```python
from build123d import *

# Parameters (mm, degrees)
SKETCH1_W           = 60
SKETCH1_H           = 65
BOSS_EXTRUDE1_DEPTH = 21
SKETCH2_W           = 60
SKETCH2_H           = 50
BOSS_EXTRUDE2_DEPTH = 15.25
FILLET1_R           = 5
SKETCH3_R           = 3.25
SKETCH3_R_2         = 1.7
CUT_EXTRUDE4_DEPTH  = 15.25
SKETCH10_R          = 1.7
CUT_EXTRUDE5_DEPTH  = 21


with BuildPart() as part:
    # Sketch1 → Boss-Extrude1 (new body)
    with BuildSketch(Plane.XY):
        with Locations((-22.911585366, 3.368902439)):
            Rectangle(SKETCH1_W, SKETCH1_H)
    extrude(amount=BOSS_EXTRUDE1_DEPTH)

    # Sketch2 → Boss-Extrude2 (add)
    with BuildSketch(Plane.XZ.offset(29.131097561)):
        with Locations((-22.911585366, 46)):
            Rectangle(SKETCH2_W, SKETCH2_H)
    extrude(amount=-BOSS_EXTRUDE2_DEPTH)

    # Fillet1
    fillet1_edges = [part.edges().sort_by_distance(p)[0] for p in [
        (-22.911585366, -13.881097561, 21),
    ]]
    fillet(fillet1_edges, radius=FILLET1_R)

    # Sketch3 → Cut-Extrude4 (cut)
    with BuildSketch(Plane(origin=(0, -13.881097561, 0), x_dir=(1, 0, 0), z_dir=(0, 1, 0))):
        with Locations(Location((-22.911585366, -48.5, 0), (0, 0, 270))):
            Circle(SKETCH3_R)
        with Locations(Location((-11.911585366, -48.5, 0), (0, 0, 270))):
            Circle(SKETCH3_R_2)
        with Locations(Location((-22.911585366, -59.75, 0), (0, 0, 270))):
            Circle(SKETCH3_R_2)
        with Locations(Location((-33.911585366, -48.5, 0), (0, 0, 270))):
            Circle(SKETCH3_R_2)
        with Locations(Location((-22.911585366, -37.5, 0), (0, 0, 270))):
            Circle(SKETCH3_R_2)
    extrude(amount=-CUT_EXTRUDE4_DEPTH, mode=Mode.SUBTRACT)

    # Sketch10 → Cut-Extrude5 (cut)
    with BuildSketch(Plane.XY.offset(21)):
        with Locations((-2.911585366, 25.868902439)):
            Circle(SKETCH10_R)
        with Locations((-2.911585366, 1.118902439)):
            Circle(SKETCH10_R)
        with Locations((-42.911585366, 25.868902439)):
            Circle(SKETCH10_R)
        with Locations((-42.911585366, 1.118902439)):
            Circle(SKETCH10_R)
    extrude(amount=-CUT_EXTRUDE5_DEPTH, mode=Mode.SUBTRACT)


solid = part.part
```
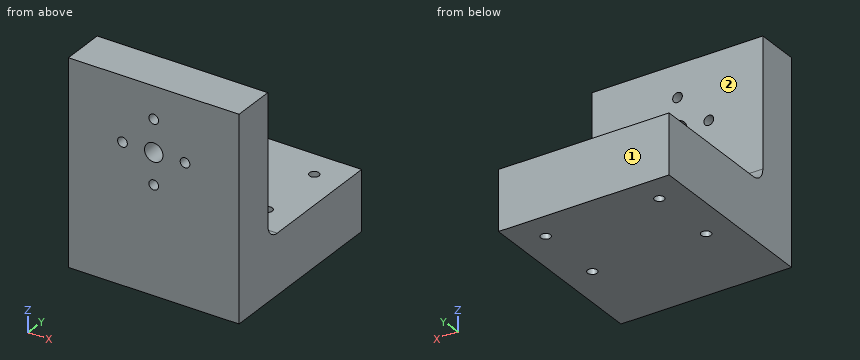
Geometry: final body of the model. Coordinates: model frame, mm. Face numbers are marked on the shaded views. A direction names the side the tool comes from. Round coordinates to 2 decimals unless told otherwise and drop trailing zeros. Loops run counter-clockwise (first coordinate to the right, second up) from the corner with the lowest first, then second, coordinate; pieces in that order, holes last. Notation, with made-up numbers: (9.25, 65.5) -> (63.25, 65.5) arc R19 cw to (63.25, 92.5) -> close; hole circle Ø5 at (36.5, 72.5). An arc over 180 degrees is marked (long way). Use one line per item in the form item = value.
Item 1: Cut plane A-A on z = 37.5. Output: boundary loops of the cut face in (x, y), then the cut area to 3 significant figures.
Evaluation:
outline = (-52.91, -29.13) -> (-24.61, -29.13) -> (-24.61, -13.88) -> (-52.91, -13.88) -> close; (-21.21, -29.13) -> (7.09, -29.13) -> (7.09, -13.88) -> (-21.21, -13.88) -> close
area = 863 mm2
Item 2: Material intervals for probe 1 along Y at (x, z) = (-43.5, 10); probe 2 along X at (y, z) = (-23, 59.75); probe 3 along Z at (x, y) = (-44.5, 9), sorted ascending.
Evaluation:
probe_1 = -29.13 to -0.48, 2.71 to 24.27, 27.46 to 35.87
probe_2 = -52.91 to -24.61, -21.21 to 7.09
probe_3 = 0 to 21
Item 3: Access query for the marked faces 1 and 2. Directions: +Z, -Z, +X, -X, +Y, -Y. A direction counts if a zero-diameter tool reaches every point of the face in a straight line with its end or side. Return the directions, or none.
Evaluation:
face_1 = +Z, -Z, +X, -X, +Y
face_2 = +Z, +X, -X, +Y
Item 4: Cut plane C-C on x = -3.5. Output: boundary loops of the cut face in (y, z).
Evaluation:
outline = (-29.13, 0) -> (-0.48, 0) -> (-0.48, 21) -> (-8.88, 21) arc R5 cw to (-13.88, 26) -> (-13.88, 71) -> (-29.13, 71) -> close; (2.71, 0) -> (24.27, 0) -> (24.27, 21) -> (2.71, 21) -> close; (27.46, 0) -> (35.87, 0) -> (35.87, 21) -> (27.46, 21) -> close
Item 5: Cut plane D-D on y = -24. Output: boundary loops of the cut face in (x, z), then the cut area to 3 significant figures.
Evaluation:
outline = (-52.91, 0) -> (7.09, 0) -> (7.09, 71) -> (-52.91, 71) -> close; hole circle Ø3.4 at (-33.91, 48.5); hole circle Ø6.5 at (-22.91, 48.5); hole circle Ø3.4 at (-22.91, 37.5); hole circle Ø3.4 at (-22.91, 59.75); hole circle Ø3.4 at (-11.91, 48.5)
area = 4,190 mm2
Item 6: Cut plane B-B on z = 48.5. Output: boundary loops of the cut face in (x, y), then the cut area to 3 significant figures.
Evaluation:
outline = (-52.91, -29.13) -> (-35.61, -29.13) -> (-35.61, -13.88) -> (-52.91, -13.88) -> close; (-32.21, -29.13) -> (-26.16, -29.13) -> (-26.16, -13.88) -> (-32.21, -13.88) -> close; (-19.66, -29.13) -> (-13.61, -29.13) -> (-13.61, -13.88) -> (-19.66, -13.88) -> close; (-10.21, -29.13) -> (7.09, -29.13) -> (7.09, -13.88) -> (-10.21, -13.88) -> close
area = 712 mm2
Item 7: Contact query for flat-ended pins moving along their axis: pin 1 Ø13.5 at (x, z) = (-33.5, 52.5) entering from +Y; pin 2 Ø4.5 at (x, y) = (-42.91, 25.87) entering from +Z; pin 3 Ø12 at (x, y) = (-40, 26) entering from -Z; pin 4 Ø2 at (x, z) = (-33.91, 48.5) entering from -Y. Output: stop coordinate, or through.
Evaluation:
pin_1 = -13.88
pin_2 = 21
pin_3 = 0
pin_4 = through
